Autodesk Inventor part; units mm, degrees
ref_plane "工作平面2" through (0, 0, 6) normal (0, 0, 1) x (1, 0, 0)
ref_plane "YZ Plane" through (0, 0, 0) normal (1, 0, 0) x (0, 1, 0)
ref_plane "XZ Plane" through (0, 0, 0) normal (0, 1, 0) x (-1, 0, 0)
sketch "草圖1" plane through (0, 0, 0) normal (0, 0, 1) x (1, 0, 0)
  line L0 (-12, 0) -> (72, 0) construction
  line L1 (0, -14) -> (0, 84) construction
  line L2 (0, 0) -> (60, 0)
  line L3 (0, 70) -> (0, 0)
  line L4 (0, 70) -> (60, 0)
  dimension "d0" = 60
  dimension "d1" = 70
extrude "擠出1" add sketch "草圖1" along normal mid plane 50
ref_plane "工作平面1" through (0, 0, 2) normal (0, 0, 1) x (1, 0, 0)
ref_plane "工作平面2" through (0, 0, 6) normal (0, 0, 1) x (1, 0, 0)
sketch "草圖3" plane through (0, 0, 6) normal (0, 0, 1) x (1, 0, 0)
  line L0 (0, 0) -> (0, 70) construction
  line L1 (0, 70) -> (60, 0) construction
  line L2 (60, 0) -> (0, 0)
  line L3 (59.7826, 0.1) -> (0.1, 69.7297)
  line L4 (0.1, 69.7297) -> (0.1, 0.1)
  line L5 (0.1, 0.1) -> (59.7826, 0.1)
  line L6 (0, 0) -> (0, 70)
  line L7 (0, 70) -> (60, 0)
  line L8 (60, 0) -> (0, 0)
  dimension "d7" = 0.1
extrude "擠出2" cut sketch "草圖3" along normal blind 10
mirror "鏡射1" about plane through (0, 0, 0) normal (0, 0, 1) of "擠出2"
properties part number "三明治"
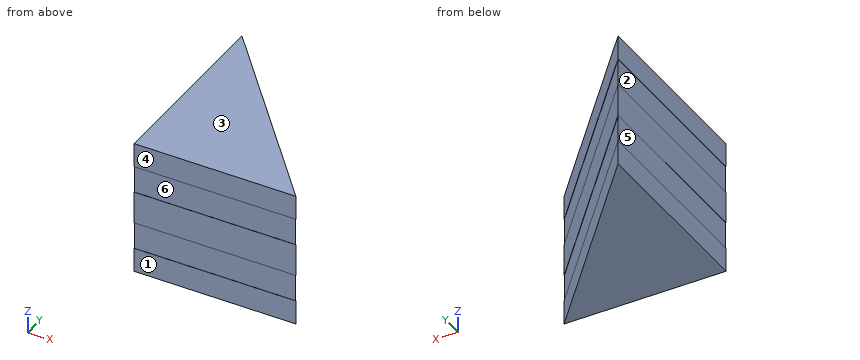
Work out the finished part from the listing and answer in its coordinate system (mm). Face numbers are marked on the shaded views. A direction names the side the tool comes from. Give positions to 0.01 mm unless a question says otherwise; leave off trailing zeros. Write each loop counter-clockwise with the first axis right and the second up, starting at its lowest first coordinate (ties: lowest second). Pieces come first, ordered by that corner, then holes.
Q1. The part is cut by section D-D on z = 7. Give the vertices of the cut face in (x, y), and give its area (3 significant figures).
Answer:
outline: (0.1, 0.1) - (59.78, 0.1) - (0.1, 69.73) - close
area: 2,080 mm2
Q2. For a pull along Z with two mould halves and no side action, classify the marked faces 1, 2 and 3 as released by +Z, released by -Z, zero draft, split by the parting line, or undercut.
Answer:
face 1: zero draft
face 2: undercut
face 3: released by +Z
Q3. Straight lines are drawn through the part: L1, parallel to X at y = 12, z = 21.5; L2, parallel to Y at x = 44, z = -5; L3, parallel to Y at x = 41, z = -0.5. For each, find the intervals that lie inside material, in ascending order.
Answer:
L1: x = 0 to 49.71
L2: y = 0 to 18.67
L3: y = 0 to 22.17
Q4. A tool of negligible diameter and unlimited length cuts with its end or side. For the marked faces 4, 5 and 6, from which of +Z, -Z, +X, -X, +Y, -Y can it reach the whole face along a straight path? Write none if from no direction.
Answer:
face 4: +Z, -Z, +X, -X, -Y
face 5: -X, +Y, -Y
face 6: +X, -X, -Y
Q5. The part is cut by section C-C on z = 1.5. Give the vertices of the cut face in (x, y), and give its area (3 significant figures).
Answer:
outline: (0, 0) - (60, 0) - (0, 70) - close
area: 2,100 mm2
Q6. Given pin 1 (6 mm diameter, centred on x = 37, z = -4, fed in from +Y); pin 2 (1 mm diameter, centred on x = 11, z = -10, fed in from +Y); pin 3 (3 mm diameter, centred on x = 43, z = 9.5, fed in from -Y), each flat-ended and moving along its own axis, determine where each tip first touches the part or whether it passes through.
Answer:
pin 1: stops at y = 30.33
pin 2: stops at y = 57.6
pin 3: stops at y = 0.1
Q7. The part is cut by section B-B on x = 30.5. Give the vertices of the cut face in (y, z).
Answer:
outline: (0, -25) - (34.42, -25) - (34.42, -16) - (34.26, -16) - (34.26, -6) - (34.42, -6) - (34.42, 6) - (34.26, 6) - (34.26, 16) - (34.42, 16) - (34.42, 25) - (0, 25) - (0, 16) - (0.1, 16) - (0.1, 6) - (0, 6) - (0, -6) - (0.1, -6) - (0.1, -16) - (0, -16) - close
Q8. The part is cut by section A-A on y = 64.5. Give the vertices of the cut face in (x, z), and give its area (3 significant figures).
Answer:
outline: (0, -25) - (4.71, -25) - (4.71, -16) - (4.58, -16) - (4.58, -6) - (4.71, -6) - (4.71, 6) - (4.58, 6) - (4.58, 16) - (4.71, 16) - (4.71, 25) - (0, 25) - (0, 16) - (0.1, 16) - (0.1, 6) - (0, 6) - (0, -6) - (0.1, -6) - (0.1, -16) - (0, -16) - close
area: 231 mm2
